```python
from build123d import *

# Parameters (mm, degrees)
CROQUIS1_R              = 1.5
SALIENTE_EXTRUIR1_DEPTH = 4
CROQUIS2_W              = 6
CROQUIS2_H              = 8
SALIENTE_EXTRUIR2_DEPTH = 23
CROQUIS3_R              = 1.5
SALIENTE_EXTRUIR3_DEPTH = 4


with BuildPart() as part:
    # Croquis1 → Saliente-Extruir1 (new body)
    with BuildSketch(Plane(origin=(0, 0, 0), x_dir=(0, 0, -1), z_dir=(1, 0, 0))):
        with BuildLine():
            Line((-29.5, 4), (29.5, 4))
            ThreePointArc((29.5, 4), (33.5, 0), (29.5, -4))
            Line((29.5, -4), (-29.5, -4))
            ThreePointArc((-29.5, -4), (-33.5, 0), (-29.5, 4))
        make_face()
        with Locations((-29.5, 0)):
            Circle(CROQUIS1_R, mode=Mode.SUBTRACT)
        with Locations((29.5, 0)):
            Circle(CROQUIS1_R, mode=Mode.SUBTRACT)
    extrude(amount=SALIENTE_EXTRUIR1_DEPTH)

    # Croquis2 → Saliente-Extruir2 (add, symmetric)
    with BuildSketch(Plane.XY):
        with Locations((7, 0)):
            Rectangle(CROQUIS2_W, CROQUIS2_H)
    extrude(amount=SALIENTE_EXTRUIR2_DEPTH, both=True)

    # Croquis3 → Saliente-Extruir3 (add)
    with BuildSketch(Plane(origin=(10, 0, 0), x_dir=(0, 0, -1), z_dir=(1, 0, 0))):
        with BuildLine():
            Line((-29.5, 4), (29.5, 4))
            ThreePointArc((29.5, 4), (33.5, 0), (29.5, -4))
            Line((29.5, -4), (-29.5, -4))
            ThreePointArc((-29.5, -4), (-33.5, 0), (-29.5, 4))
        make_face()
        with Locations((-29.5, 0)):
            Circle(CROQUIS3_R, mode=Mode.SUBTRACT)
        with Locations((29.5, 0)):
            Circle(CROQUIS3_R, mode=Mode.SUBTRACT)
    extrude(amount=SALIENTE_EXTRUIR3_DEPTH)


solid = part.part
```
Here's how the part is built. I have some questions about the finished solid (model axes, mm). A direction names the side the tool comes from. Round coordinates to 2 decimals unless told otherwise and drop trailing zeros. Order: outer loops, then holes, each group sorted by start corner. A loop starts at its lowest first (then second) coordinate and runs counter-clockwise, first axis right, second up. Notation, with made-up numbers: M 17,14.25 L 31,14.25 A16 ccw 31,26.25 Z; hole C 36.25,28 d3. An arc over 180 degrees is marked long. Use CSV: the item, a comma, the result in double quotes.
1) I want a section at A-A (x = 2). List the corners of the cut face in (y, z) for me.
Taken from the geometry:
outline,"M -4,-29.5 A4 ccw 4,-29.5 L 4,29.5 A4 ccw -4,29.5 Z; hole C 0,-29.5 d3; hole C 0,29.5 d3"
2) On a 3-axis mill with a long thin cutter (end or side, diameter ignored), from which of +Z, -Z, +X, -X, +Y, -Y can I reach the whole of each face in a straight line? I mean faces 1 (the flat face through (7, 0, 23)), 2 (the flat face through (10, 0, -27)), 3 (the cylindrical face through (12, -0.1, 33.5)). Say none if no direction works.
Taken from the geometry:
face 1,"+Z, +Y, -Y"
face 2,"-Z, +Y, -Y"
face 3,"+Z, +X, -X"
3) I need wall thicknesses on line 1 along X through (y, z) = (1.5, -25); line 2 along Y through (x, z) = (2.5, 29.5); line 3 along Z through (x, y) = (7.25, -0.5). Which ranges of each line are inside material? Lowest first, please. Write a range as [from, to].
Taken from the geometry:
line 1,"[0, 4], [10, 14]"
line 2,"[-4, -1.5], [1.5, 4]"
line 3,"[-23, 23]"
4) I'm going to push flat-ended pins straight in: P1, Ø3, axis at x = 7.5, y = -2, coming from the -Z side; P2, Ø2, axis at x = 1.5, y = 3, coming from the -Z side; P3, Ø1, axis at x = 12, y = -2, coming from the -Z side. Where does each tip first touch, or does it pass through?
Taken from the geometry:
P1,"z = -23"
P2,"z = -32.96"
P3,"z = -33.21"
5) If we mould it in two halves opening along X, with no side actions, what happens to faces 4 (the flat face through (14, 0, 0)), 5 (the cylindrical face through (12, 0, -28)), 6 (the flat face through (4, 0, -27)), 7 (the flat face through (4, 0, 27))? For each: pulls with the +X half, pulls with the -X half, needs draft (parallel to the pull), parting line crosses it, or undercut.
Taken from the geometry:
face 4,"pulls with the +X half"
face 5,"needs draft"
face 6,"undercut"
face 7,"undercut"
6) I want a section at C-C (x = 7.25). List the corners of the cut face in (y, z) for me, then the cut area to 3 significant figures.
Taken from the geometry:
outline,"M -4,-23 L 4,-23 L 4,23 L -4,23 Z"
area,"368 mm^2"
7) I want a section at B-B (y = 2.75). List the corners of the cut face in (x, z) for me, then the cut area to 3 significant figures.
Taken from the geometry:
outline,"M 0,-32.4 L 4,-32.4 L 4,-23 L 10,-23 L 10,-32.4 L 14,-32.4 L 14,32.4 L 10,32.4 L 10,23 L 4,23 L 4,32.4 L 0,32.4 Z"
area,"794 mm^2"
8) I want a section at D-D (y = -3). List the corners of the cut face in (x, z) for me, then the cut area to 3 significant figures.
Taken from the geometry:
outline,"M 0,-32.15 L 4,-32.15 L 4,-23 L 10,-23 L 10,-32.15 L 14,-32.15 L 14,32.15 L 10,32.15 L 10,23 L 4,23 L 4,32.15 L 0,32.15 Z"
area,"790 mm^2"
